Check sheet for the modelled part. Datum: model origin and axes. Units: mm. A direction names the side the tool comes from. Round coordinates to 2 decimals unless told otherwise and drop trailing zeros. Order: outer loops, then holes, each group sorted by start corner. A loop starts at its lowest first (then second) coordinate and runs counter-clockwise, first axis right, second up. Notation, with made-up numbers: M 59.25,85 L 72.25,85 A27 cw 72.25,123 Z; hole C 45,20.25 d7. An arc over 180 degrees is marked long. One line per item, written item: value. Start each with the question number.
(1) Release check for a two-part mould opening along X. For faces 1 (the face through (-22.5, 21.3, 4.6)), 2 (the face through (0, 30, 5)), 3 (the face through (-15, 3, 24.65)) record: released by +X, released by -X, zero draft, split by the parting line, or undercut.
(2) Cross-section at B-B, the plane x = -1. Enter the section's corners in (y, z).
(3) Thickness scan on L1, parallel to Y at x = 1, z = 1.75; L2, parallel to X at y = 37, z = 1.5; L3, parallel to Z at x = -7.5, y = 20.5. Record the ranges inside material, lowest first.
(4) Cross-section at C-C, the plane z = 2.5. Enter the section's corners in (x, y), and give its area (3 significant figures).
(5) Cross-section at A-A, the plane y = 48.5. Enter the section's corners in (x, z), and give its area (3 significant figures).
(6) Cross-section at D-D, the plane x = 10. Enter the section's corners in (y, z).
(7) Access from +Z, -Z, +X, -X, +Y, -Y to the whole of each face (thin tool, end or side, straight path). Record for faces 4 (the face through (-12.43, 2.54, 24.2)), 5 (the face through (0, 0, 2)), 6 (the face through (0, 5, 16)), 7 (the face through (-12.43, 24.2, 2.54)).
(8) Depth check by flat-ended pin: pin 1 Ø8 at (x, z) = (-8, 18) entering from -Y; pin 2 Ø3 at (x, y) = (17.5, 31) entering from +Z; pin 3 Ø10 at (x, y) = (-16.5, 48.5) entering from -Z; pin 4 Ø12 at (x, z) = (-4.5, 8.5) entering from -Y. Enter the tip coordinate at first touch or a pass-through.
from build123d import *

# Parameters (mm, degrees)
BOX016_W      = 6
BOX016_H      = 10
BOX016_DEPTH  = 3.3
FILLET001_R   = 1.5
BOX013_W      = 6
BOX013_H      = 3.3
BOX013_DEPTH  = 10
FILLET003_R   = 1.5
BOX015_W      = 6
BOX015_H      = 10
BOX015_DEPTH  = 3.3
FILLET002_1_R = 1.5
FILLET002_2_R = 1
BOX012_W      = 16
BOX012_H      = 25
BOX012_DEPTH  = 6
BOX017_W      = 45
BOX017_H      = 50
BOX017_DEPTH  = 23
BOX014_W      = 6
BOX014_H      = 3.3
BOX014_DEPTH  = 10
FILLET_R      = 1.5
BOX009_W      = 16
BOX009_H      = 50
BOX009_DEPTH  = 4
BOX_W         = 45
BOX_H         = 55
BOX_DEPTH     = 28
BOX007_W      = 25
BOX007_H      = 8
BOX007_DEPTH  = 8


with BuildPart() as fillet001:
    # Box016 → Box016 (new body)
    with BuildSketch(Plane(origin=(-18, 0, 21.35), x_dir=(1, 0, 0), z_dir=(0, 0, 1))):
        with Locations((3, 5)):
            Rectangle(BOX016_W, BOX016_H)
    extrude(amount=BOX016_DEPTH)

    # Fillet001
    fillet001_edges = [fillet001.edges().sort_by_distance(p)[0] for p in [
        (-18, 5, 24.65),
        (-18, 5, 21.35),
        (-12, 5, 24.65),
        (-12, 5, 21.35),
    ]]
    fillet(fillet001_edges, radius=FILLET001_R)


with BuildPart() as fillet003:
    # Box013 → Box013 (new body)
    with BuildSketch(Plane(origin=(12, 21.35, 0), x_dir=(1, 0, 0), z_dir=(0, 0, 1))):
        with Locations((3, 1.65)):
            Rectangle(BOX013_W, BOX013_H)
    extrude(amount=BOX013_DEPTH)

    # Fillet003
    fillet003_edges = [fillet003.edges().sort_by_distance(p)[0] for p in [
        (12, 21.35, 5),
        (12, 24.65, 5),
        (18, 21.35, 5),
        (18, 24.65, 5),
    ]]
    fillet(fillet003_edges, radius=FILLET003_R)


with BuildPart() as fillet002:
    # Box015 → Box015 (new body)
    with BuildSketch(Plane(origin=(12, 0, 21.35), x_dir=(1, 0, 0), z_dir=(0, 0, 1))):
        with Locations((3, 5)):
            Rectangle(BOX015_W, BOX015_H)
    extrude(amount=BOX015_DEPTH)

    # Fillet002 1
    fillet002_1_edges = [fillet002.edges().sort_by_distance(p)[0] for p in [
        (12, 5, 21.35),
        (18, 5, 24.65),
        (18, 5, 21.35),
    ]]
    fillet(fillet002_1_edges, radius=FILLET002_1_R)

    # Fillet002 2
    fillet002_2_edges = [fillet002.edges().sort_by_distance(p)[0] for p in [
        (12, 5, 24.65),
    ]]
    fillet(fillet002_2_edges, radius=FILLET002_2_R)


with BuildPart() as box012:
    # Box012 → Box012 (new body)
    with BuildSketch(Plane(origin=(-8, 35, 4), x_dir=(1, 0, 0), z_dir=(0, 0, 1))):
        with Locations((8, 12.5)):
            Rectangle(BOX012_W, BOX012_H)
    extrude(amount=BOX012_DEPTH)


with BuildPart() as box017:
    # Box017 → Box017 (new body)
    with BuildSketch(Plane(origin=(-22.5, 5, 5), x_dir=(1, 0, 0), z_dir=(0, 0, 1))):
        with Locations((22.5, 25)):
            Rectangle(BOX017_W, BOX017_H)
    extrude(amount=BOX017_DEPTH)


with BuildPart() as fillet_body:
    # Box014 → Box014 (new body)
    with BuildSketch(Plane(origin=(-18, 21.35, 0), x_dir=(1, 0, 0), z_dir=(0, 0, 1))):
        with Locations((3, 1.65)):
            Rectangle(BOX014_W, BOX014_H)
    extrude(amount=BOX014_DEPTH)

    # Fillet
    fillet_edges = [fillet_body.edges().sort_by_distance(p)[0] for p in [
        (-18, 21.35, 5),
        (-18, 24.65, 5),
        (-12, 21.35, 5),
        (-12, 24.65, 5),
    ]]
    fillet(fillet_edges, radius=FILLET_R)


with BuildPart() as fusion001:
    # Box009 → Box009 (new body)
    with BuildSketch(Plane(origin=(-8, 0, 0), x_dir=(1, 0, 0), z_dir=(0, 0, 1))):
        with Locations((8, 25)):
            Rectangle(BOX009_W, BOX009_H)
    extrude(amount=BOX009_DEPTH)

    # Fusion001: union Fillet001, Fillet003, Fillet002, Box012, Box017, Fillet body
    add(fillet001.part)
    add(fillet003.part)
    add(fillet002.part)
    add(box012.part)
    add(box017.part)
    add(fillet_body.part)


with BuildPart() as box:
    # Box → Box (new body)
    with BuildSketch(Plane(origin=(-22.5, 0, 0), x_dir=(1, 0, 0), z_dir=(0, 0, 1))):
        with Locations((22.5, 27.5)):
            Rectangle(BOX_W, BOX_H)
    extrude(amount=BOX_DEPTH)


with BuildPart() as cut:
    # Box007 → Box007 (new body)
    with BuildSketch(Plane(origin=(-12.5, -1, -1), x_dir=(1, 0, 0), z_dir=(0, 0, 1))):
        with Locations((12.5, 4)):
            Rectangle(BOX007_W, BOX007_H)
    extrude(amount=BOX007_DEPTH)

    # Fusion: union Box
    add(box.part)

    # Cut: cut Fusion001
    add(fusion001.part, mode=Mode.SUBTRACT)


solid = cut.part
Values found:
1. face 1: released by -X
1. face 2: zero draft
1. face 3: undercut
2. outline: M -1,-1 L 7,-1 L 7,0 L 0,0 L 0,4 L 35,4 L 35,5 L 5,5 L 5,28 L 0,28 L 0,7 L -1,7 Z; M 50,0 L 55,0 L 55,4 L 50,4 Z
3. L1: -1 to 0, 50 to 55
3. L2: -22.5 to -8, 8 to 22.5
3. L3: 4 to 5
4. outline: M -22.5,0 L -12.5,0 L -12.5,-1 L 12.5,-1 L 12.5,0 L 22.5,0 L 22.5,55 L -22.5,55 Z; hole M -18,22.85 A1.5 ccw -16.5,21.35 L -13.5,21.35 A1.5 ccw -12,22.85 L -12,23.15 A1.5 ccw -13.5,24.65 L -16.5,24.65 A1.5 ccw -18,23.15 Z; hole M -8,0 L 8,0 L 8,50 L -8,50 Z; hole M 12,22.85 A1.5 ccw 13.5,21.35 L 16.5,21.35 A1.5 ccw 18,22.85 L 18,23.15 A1.5 ccw 16.5,24.65 L 13.5,24.65 A1.5 ccw 12,23.15 Z
4. area: 1,660 mm^2
5. outline: M -22.5,0 L -8,0 L -8,5 L -22.5,5 Z; M 8,0 L 22.5,0 L 22.5,5 L 8,5 Z
5. area: 145 mm^2
6. outline: M -1,-1 L 7,-1 L 7,0 L 55,0 L 55,5 L 5,5 L 5,28 L 0,28 L 0,7 L -1,7 Z
7. face 4: +Y, -Y
7. face 5: none
7. face 6: +Z, +X, -X, +Y
7. face 7: +Z, -Z
8. pin 1: y = 0
8. pin 2: z = 5
8. pin 3: z = 0
8. pin 4: y = -1
